Can you work these out from the model? Positions are in its coordinate system, mm. A direction names the side the tool comes from. Coordinates: 2 decimals unless noted, no trailing zeros. Order: outer loops, then holes, each group sorted by start corner. A loop starts at its lowest first (then second) coordinate and runs counter-clockwise, first axis right, second up.
```python
from build123d import *

# Parameters (mm, degrees)
F0_W     = 95.25
F0_H     = 7.9375
F0_R     = 2.38125
F1_DEPTH = 3.175
F2_DEPTH = 4.7625
F3_T     = -1.5875
F4_R     = 1.5875
F4_R_2   = 0.79375
F5_DEPTH = 1.5875


# Not quite as in the source:
# - a feature names something its author has since deleted; it is built from what else it names


with BuildPart() as f1:
    # F0 (on Top) → F1 (new body)
    with BuildSketch(Plane.XY):
        Rectangle(F0_W, F0_H)
        with Locations((-43.65625, 0)):
            Circle(F0_R, mode=Mode.SUBTRACT)
        with Locations((-35.71875, 0)):
            Circle(F0_R, mode=Mode.SUBTRACT)
        with Locations((-27.78125, 0)):
            Circle(F0_R, mode=Mode.SUBTRACT)
        with Locations((-19.84375, 0)):
            Circle(F0_R, mode=Mode.SUBTRACT)
        with Locations((-11.90625, 0)):
            Circle(F0_R, mode=Mode.SUBTRACT)
        with Locations((-3.96875, 0)):
            Circle(F0_R, mode=Mode.SUBTRACT)
        with Locations((3.96875, 0)):
            Circle(F0_R, mode=Mode.SUBTRACT)
        with Locations((11.90625, 0)):
            Circle(F0_R, mode=Mode.SUBTRACT)
        with Locations((19.84375, 0)):
            Circle(F0_R, mode=Mode.SUBTRACT)
        with Locations((27.78125, 0)):
            Circle(F0_R, mode=Mode.SUBTRACT)
        with Locations((35.71875, 0)):
            Circle(F0_R, mode=Mode.SUBTRACT)
        with Locations((43.65625, 0)):
            Circle(F0_R, mode=Mode.SUBTRACT)
    extrude(amount=F1_DEPTH)

    # F0 (on Top) → F2 (join)
    with BuildSketch(Plane.XY):
        with Locations((-43.65625, 0)):
            Circle(F0_R)
        with Locations((-27.78125, 0)):
            Circle(F0_R)
        with Locations((-35.71875, 0)):
            Circle(F0_R)
        with Locations((-19.84375, 0)):
            Circle(F0_R)
        with Locations((-11.90625, 0)):
            Circle(F0_R)
        with Locations((-3.96875, 0)):
            Circle(F0_R)
        with Locations((3.96875, 0)):
            Circle(F0_R)
        with Locations((11.90625, 0)):
            Circle(F0_R)
        with Locations((19.84375, 0)):
            Circle(F0_R)
        with Locations((27.78125, 0)):
            Circle(F0_R)
        with Locations((35.71875, 0)):
            Circle(F0_R)
        with Locations((43.65625, 0)):
            Circle(F0_R)
    extrude(amount=F2_DEPTH)

    # F3
    f3_openings = [f1.faces().sort_by_distance(p)[0] for p in [
        (0, 0, 0),
    ]]
    offset(amount=F3_T, openings=f3_openings, kind=Kind.INTERSECTION)

    # F4 (on face) → F5 (join)
    with BuildSketch(Plane(origin=(0, 0, 1.5875), x_dir=(1, 0, 0), z_dir=(0, 0, -1))):
        with Locations((-39.6875, 0)):
            Circle(F4_R)
        with Locations((-39.6875, 0)):
            Circle(F4_R_2, mode=Mode.SUBTRACT)
        with Locations((-31.75, 0)):
            Circle(F4_R)
        with Locations((-31.75, 0)):
            Circle(F4_R_2, mode=Mode.SUBTRACT)
        with Locations((-23.8125, 0)):
            Circle(F4_R)
        with Locations((-23.8125, 0)):
            Circle(F4_R_2, mode=Mode.SUBTRACT)
        with Locations((-15.875, 0)):
            Circle(F4_R)
        with Locations((-15.875, 0)):
            Circle(F4_R_2, mode=Mode.SUBTRACT)
        with Locations((-7.9375, 0)):
            Circle(F4_R)
        with Locations((-7.9375, 0)):
            Circle(F4_R_2, mode=Mode.SUBTRACT)
        Circle(F4_R)
        Circle(F4_R_2, mode=Mode.SUBTRACT)
        with Locations((7.9375, 0)):
            Circle(F4_R)
        with Locations((7.9375, 0)):
            Circle(F4_R_2, mode=Mode.SUBTRACT)
        with Locations((15.875, 0)):
            Circle(F4_R)
        with Locations((15.875, 0)):
            Circle(F4_R_2, mode=Mode.SUBTRACT)
        with Locations((23.8125, 0)):
            Circle(F4_R)
        with Locations((23.8125, 0)):
            Circle(F4_R_2, mode=Mode.SUBTRACT)
        with Locations((31.75, 0)):
            Circle(F4_R)
        with Locations((31.75, 0)):
            Circle(F4_R_2, mode=Mode.SUBTRACT)
        with Locations((39.6875, 0)):
            Circle(F4_R)
        with Locations((39.6875, 0)):
            Circle(F4_R_2, mode=Mode.SUBTRACT)
    extrude(amount=F5_DEPTH)


solid = f1.part
```
1. Please list where these lines run through material, in increasing order: probe 1 along Y at (x, z) = (31.75, 0.6); probe 2 along Y at (x, z) = (-12, 3.1); probe 3 along Y at (x, z) = (-14.5, 0.6).
Completed:
probe 1: y = -3.97 to -2.38, -1.59 to -0.79, 0.79 to 1.59, 2.38 to 3.97
probe 2: y = -3.97 to -0.79, 0.79 to 3.97
probe 3: y = -3.97 to -2.38, -0.79 to 0.79, 2.38 to 3.97
2. Imagine slicing it at B-B on x = -31.75. Please give me the cut outline in (y, z) (1 decimal), then the cut area to 3 significant figures.
Completed:
outline: (-4, 0) - (-2.4, 0) - (-2.4, 1.6) - (-1.6, 1.6) - (-1.6, 0) - (-0.8, 0) - (-0.8, 1.6) - (0.8, 1.6) - (0.8, 0) - (1.6, 0) - (1.6, 1.6) - (2.4, 1.6) - (2.4, 0) - (4, 0) - (4, 3.2) - (-4, 3.2) - close
area: 20.2 mm2
3. On a 3-axis mill with a long thin cutter (end or side, diameter ignored), from which of +Z, -Z, +X, -X, +Y, -Y can I reach the whole of each face in a straight line? I mean faces 4 (the flat face through (40, -1, 0)), 5 (the cylindrical face through (-30.236, -0.477, 0.805)), 6 (the cylindrical face through (-22.223, 0.105, 3.958)). Say none if no direction works.
Completed:
face 4: -Z, +X, -X, +Y, -Y
face 5: -Z
face 6: +Z
4. I'm going to push flat-ended pins straight in: pin 1 (1.4 mm diameter, centred on x = -23.81, y = 0, fed in from -Z); pin 2 (2.5 mm diameter, centred on x = 7.94, y = 0, fed in from +Z) (3 decimals). Where does each tip first touch, or does it pass through?
Completed:
pin 1: stops at z = 1.59
pin 2: stops at z = 3.175
5. Thinking about a two-plate mould opening in Y: for faces 1 (the flat face through (4, 0, 4.762)), 2 (the cylindrical face through (9.527, 0.105, 3.958)), 3 (the cylindrical face through (4.726, 0.238, 2.37)), which applies, pulls with the +Y half, pulls with the -Y half, needs draft (parallel to the pull), parting line crosses it, or undercut?
Completed:
face 1: needs draft
face 2: parting line crosses it
face 3: undercut
6. Imagine slicing it at A-A on z = 3.9. Give the number of separate pieces and of enclosed holes in the cut face, then the cut area to 3 significant figures.
Completed:
separate pieces: 12
enclosed holes: 0
area: 214 mm2
